Autodesk Inventor part; units mm, degrees
ref_plane "YZ Plane" through (0, 0, 0) normal (1, 0, 0) x (0, 1, 0)
ref_plane "XZ Plane" through (0, 0, 0) normal (0, 1, 0) x (-1, 0, 0)
ref_plane "XY Plane" through (0, 0, 0) normal (0, 0, 1) x (1, 0, 0)
sketch "Sketch1" plane through (0, 0, 0) normal (0, 0, 1) x (1, 0, 0)
  line L0 (-8, -10) -> (8, -10)
  line L1 (8, -10) -> (8, 10)
  line L2 (8, 10) -> (-8, 10)
  line L3 (-8, 10) -> (-8, -10)
  line L4 (-8, -10) -> (8, 10) construction
  line L5 (8, -10) -> (-8, 10) construction
  point P0 (0, 0)
  dimension "d0" = 16
  dimension "d1" = 20
extrude "Plate1" add sketch "Sketch1" along normal blind 1.2
sketch "Sketch2" plane through (6.8, 10, 0) normal (1, 0, 0) x (0, 1, 0)
  line L0 (-20, 0) -> (0, 0)
  line L1 (0, 0) -> (0, 16)
  line L2 (0, 16) -> (-20, 16)
  line L3 (-20, 16) -> (-20, 0)
edge flange "Flange1" height 16 angle 90 thickness 1.2 bend radius 1.2 thickness toward (1, 0, 0) relief tear relief width 1.2 relief depth 0.6 edges at (8, 0, 1.2) wall of the first edge with corners at (6.8, -10, 0) (6.8, 10, 0) (6.8, 10, 16) (6.8, -10, 16)
bend "Bend1"
corner "Corner1"
chamfer "Corner Chamfer1" distance 3 angle 45 4 edges at (-8, 10, 0.6) (-8, -10, 0.6) (7.4, -10, 16) (7.4, 10, 16)
sketch "Sketch3" plane through (6.8, -10, 2.4) normal (-1, 0, 0) x (0, 0, 1)
  line L0 (13.6, 3) -> (13.6, 17)
  line L1 (-2.4, 17) -> (-2.4, 3)
  point P0 (-2.4, 10)
  point P1 (7.6, 10)
  point P2 (-2.4, 10)
  dimension "d16" = 6
hole "Hole1" at (6.8, 0, 10) direction (1, 0, 0) diameter 3 depth 1.2 tip angle 118
sketch "Sketch4" plane through (0, 0, 1.2) normal (0, 0, 1) x (1, 0, 0)
  circle A0 centre (-0.5392, 0) radius 2.1 construction
  circle A1 centre (-0.5392, 0) radius 2.5
  point P0 (0, 0)
  dimension "d24" = 0.4
extrude "Cut1" cut sketch "Sketch4" against normal blind 1.2
equation "\"d22\" = Thickness"
equation "\"d25\" = Thickness"
equation "\"d3\" = BendReliefWidth"
equation "\"d4\" = BendReliefDepth"
equation "\"d5\" = MinimumRemnant"
equation "\"d6\" = BendRadius"
equation "\"d9\" = BendRadius"
equation "\"d10\" = CornerReliefSize"
equation "\"d11\" = GapSize"
equation "\"d12\" = JacobiRadiusSize"
equation "\"BendRadius\" = Thickness"
equation "\"BendReliefWidth\" = Thickness"
equation "\"BendReliefDepth\" = 0.5 * Thickness"
equation "\"CornerReliefSize\" = 4 * Thickness"
equation "\"MinimumRemnant\" = 2 * Thickness"
equation "\"TransitionRadius\" = BendRadius"
equation "\"JacobiRadiusSize\" = BendRadius"
equation "\"GapSize\" = Thickness"
equation "\"d2\" = BendRadius"
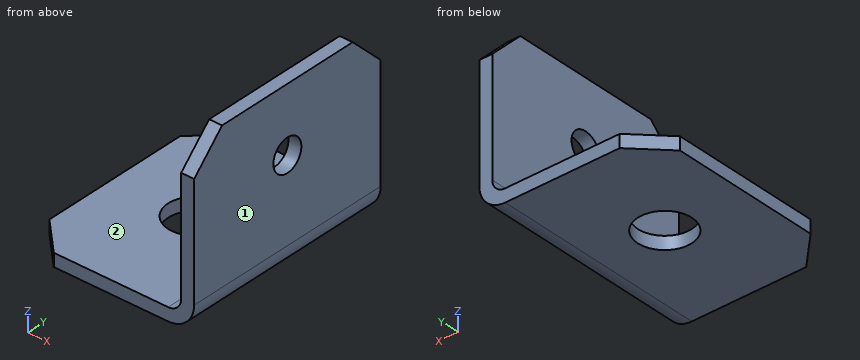
CAD build for the part. Positions are in the model's coordinates, mm. Face numbers are marked on the shaded views. A direction names the side the tool comes from. Round coordinates to 2 decimals unless told otherwise and drop trailing zeros. Loops run counter-clockwise (first coordinate to the right, second up) from the corner with the lowest first, then second, coordinate; pieces in that order, holes last.
(1) Which spindle directions (+Z, -Z, +X, -X, +Y, -Y) get a long thin tool onto all of the face, cutting with end or side? Do the marked faces 1 and 2. Say none if no direction does.
(2) Cut at C-C (x = 1.25). Give the cut face in (y, z), plus the area to 3 significant figures.
(3) Cut at D-D (x = -6.75). Give the cut face in (y, z).
(4) Cut at A-A (y = 0). Give the cut face in (x, z).
(5) Wall check: line 1 along Y through (x, z) = (7.55, 10); line 2 along X through (y, z) = (6, 7.5); line 3 along Z through (x, y) = (-5.5, 2.25). Give the ranges that are in metal, low to high.
(6) Cut at B-B (z = 10). Give the cut face in (x, y).
(7) Drop flat-ended pins along their axis: pin 1 (3 mm diameter, centred on x = -2.5, y = -5, fed in from +Z); pin 2 (4 mm diameter, centred on x = -0.54, y = 0, fed in from -Z); pin 3 (4 mm diameter, centred on y = -3.5, z = 11, fed in from -X); pin 4 (5 mm diameter, centred on y = 7.5, z = 4, fed in from -X). Give the stop position or say it passes through.
Findings below:
1. face 1: +Z, -Z, +X, +Y, -Y
1. face 2: +Z, -X, +Y, -Y
2. outline: (-10, 0) - (-1.75, 0) - (-1.75, 1.2) - (-10, 1.2) - close; (1.75, 0) - (10, 0) - (10, 1.2) - (1.75, 1.2) - close
2. area: 19.8 mm2
3. outline: (-8.25, 0) - (8.25, 0) - (8.25, 1.2) - (-8.25, 1.2) - close
4. outline: (-8, 0) - (-3.04, 0) - (-3.04, 1.2) - (-8, 1.2) - close; (1.96, 0) - (5.6, 0) arc R2.4 ccw to (8, 2.4) - (8, 8.5) - (6.8, 8.5) - (6.8, 2.4) arc R1.2 cw to (5.6, 1.2) - (1.96, 1.2) - close; (6.8, 11.5) - (8, 11.5) - (8, 16) - (6.8, 16) - close
5. line 1: y = -10 to -1.5, 1.5 to 10
5. line 2: x = 6.8 to 8
5. line 3: z = 0 to 1.2
6. outline: (6.8, -10) - (8, -10) - (8, -1.5) - (6.8, -1.5) - close; (6.8, 1.5) - (8, 1.5) - (8, 10) - (6.8, 10) - close
7. pin 1: stops at z = 1.2
7. pin 2: passes through
7. pin 3: stops at x = 6.8
7. pin 4: stops at x = 6.39
